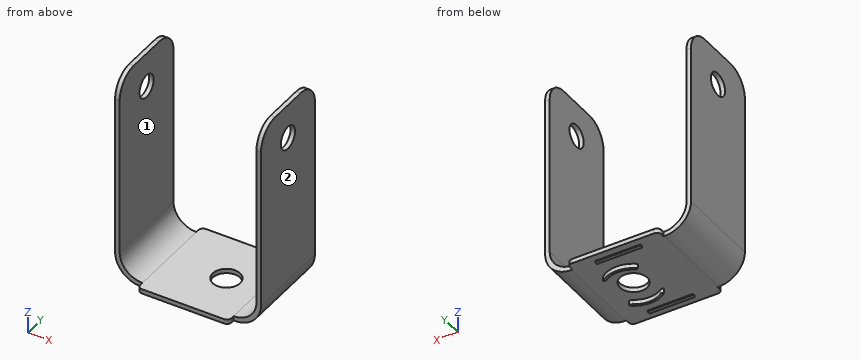
```python
from build123d import *

# Parameters (mm, degrees)
F1_DEPTH  = 38
F3_D      = 12
F5_DEPTH  = 2
F6_R      = 10
F8_DEPTH  = 0.5
F10_DEPTH = 2
F12_D     = 10


with BuildPart() as f1:
    # F0 (on Front) → F1 (new body)
    with BuildSketch(Plane.XZ):
        with BuildLine():
            Line((20, 0), (0, 0))
            Line((0, 0), (-20, 0))
            ThreePointArc((-20, 0), (-27.0710678119, 2.9289321881), (-30, 10))
            Line((-30, 10), (-30, 90))
            Line((-30, 90), (-32, 90))
            Line((-32, 90), (-32, 9.5))
            ThreePointArc((-32, 9.5), (-28.6317279836, 1.3682720164), (-20.5, -2))
            Line((-20.5, -2), (0, -2))
            Line((0, -2), (20.5, -2))
            ThreePointArc((20.5, -2), (28.6317279836, 1.3682720164), (32, 9.5))
            Line((32, 9.5), (32, 90))
            Line((32, 90), (30, 90))
            Line((30, 90), (30, 10))
            ThreePointArc((30, 10), (27.0710678119, 2.9289321881), (20, 0))
        make_face()
    extrude(amount=F1_DEPTH)

    # F3 (through all)
    with Locations(Plane.XY):
        with Locations((5, -19)):
            Hole(F3_D / 2)

    # F4 (on face) → F5 (join)
    with BuildSketch(Plane(origin=(0, 0, -2), x_dir=(1, 0, 0), z_dir=(0, 0, -1))):
        with BuildLine():
            ThreePointArc((-1, 28.2195444573), (5, 30), (11, 28.2195444573))
            ThreePointArc((11, 28.2195444573), (11.8405728739, 27.8759539642), (12.6811457479, 28.2195444573))
            ThreePointArc((12.6811457479, 28.2195444573), (5, 31), (-2.6811457479, 28.2195444573))
            ThreePointArc((-2.6811457479, 28.2195444573), (-1.8405728739, 27.8759539642), (-1, 28.2195444573))
        make_face()
        with BuildLine():
            ThreePointArc((11, 9.7804555427), (5, 8), (-1, 9.7804555427))
            ThreePointArc((-1, 9.7804555427), (-1.8405728739, 10.1240460358), (-2.6811457479, 9.7804555427))
            ThreePointArc((-2.6811457479, 9.7804555427), (5, 7), (12.6811457479, 9.7804555427))
            ThreePointArc((12.6811457479, 9.7804555427), (11.8405728739, 10.1240460358), (11, 9.7804555427))
        make_face()
    extrude(amount=F5_DEPTH)

    # F6
    f6_edges = [f1.edges().sort_by_distance(p)[0] for p in [
        (-31, -38, 90),
        (31, -38, 90),
        (-31, 0, 90),
        (31, 0, 90),
    ]]
    fillet(f6_edges, radius=F6_R)

    # F7 (on face) → F8 (join)
    with BuildSketch(Plane(origin=(0, 0, -2), x_dir=(1, 0, 0), z_dir=(0, 0, -1))):
        Polygon((10, 36.75), (10, 37.5), (10, 38.25), (-10, 38.25), (-10, 36.75), align=None)
        Polygon((10, -0.25), (10, 0.5), (10, 1.25), (-10, 1.25), (-10, -0.25), align=None)
    extrude(amount=F8_DEPTH)

    # F9 (on face) → F10 (join)
    with BuildSketch(Plane.XY):
        with BuildLine():
            Line((-20, 1.5), (-20, 0))
            Line((-20, 0), (20, 0))
            Line((20, 0), (20, 1.5))
            ThreePointArc((20, 1.5), (19.4142135624, 2.9142135624), (18, 3.5))
            Line((18, 3.5), (-18, 3.5))
            ThreePointArc((-18, 3.5), (-19.4142135624, 2.9142135624), (-20, 1.5))
        make_face()
        with BuildLine():
            ThreePointArc((18, -41.5), (19.4142135624, -40.9142135624), (20, -39.5))
            Line((20, -39.5), (20, -38))
            Line((20, -38), (-20, -38))
            Line((-20, -38), (-20, -39.5))
            ThreePointArc((-20, -39.5), (-19.4142135624, -40.9142135624), (-18, -41.5))
            Line((-18, -41.5), (18, -41.5))
        make_face()
    extrude(amount=-F10_DEPTH)

    # F12 (through all)
    with Locations(Plane.YZ.offset(32)):
        with Locations((-19, 75)):
            Hole(F12_D / 2)


solid = f1.part
```
Source: CAD feature listing. Evaluate the final solid. Frame: model axes, mm. Face numbers are marked on the shaded views. A direction names the side the tool comes from. Round coordinates to 2 decimals unless told otherwise and drop trailing zeros. Order: outer loops, then holes, each group sorted by start corner. A loop starts at its lowest first (then second) coordinate and runs counter-clockwise, first axis right, second up. Notation, with made-up numbers: (67.5, -26.5) -> (117.5, -26.5) arc R30 cw to (117.5, 8.5) -> close; hole circle Ø2 at (-18, 85.5). An arc over 180 degrees is marked (long way). One line per item, written item: value. Start each with the question number.
Q1. Section query B-B (z = 57). Return the cut outline in (x, y).
Q2. Section query C-C (x = 5). Return the cut outline in (y, z).
Q3. Section query A-A (y = -19). Return the cut outline in (x, z), plus the area to 3 significant figures.
Q4. Section query D-D (z = 75). Return the cut outline in (x, y).
Q5. Material intervals for probe 1 along X at (y, z) = (-15, 35.5); probe 2 along Z at (x, y) = (-8, -13); probe 3 along X at (y, z) = (-34.5, 1.5), sorted ascending.
Q6. Access query for the marked faces 1 and 2. Directions: +Z, -Z, +X, -X, +Y, -Y. A direction counts if a zero-diameter tool reaches every point of the face in a straight line with its end or side. Return the directions, or none.
Q7. Pin query (flat end, axial travel): pin 1 (4 mm diameter, centred on x = -4, y = -18, fed in from -Z); pin 2 (1.6 mm diameter, centred on y = -38.5, z = -0.5, fed in from -X); pin 3 (12 mm diameter, centred on x = -6.5, y = -14, fed in from +Z); pin 4 (9 mm diameter, centred on y = -19, z = 75, fed in from -X). Return the tip coordinate at first contact, or that it passes through.
Findings below:
1. outline: (-32, -38) -> (-30, -38) -> (-30, 0) -> (-32, 0) -> close; (30, -38) -> (32, -38) -> (32, 0) -> (30, 0) -> close
2. outline: (-41.5, -2) -> (-38.25, -2) -> (-38.25, -2.5) -> (-36.75, -2.5) -> (-36.75, -2) -> (-31, -2) -> (-31, -4) -> (-30, -4) -> (-30, -2) -> (-25, -2) -> (-25, 0) -> (-41.5, 0) -> close; (-13, -2) -> (-8, -2) -> (-8, -4) -> (-7, -4) -> (-7, -2) -> (-1.25, -2) -> (-1.25, -2.5) -> (0.25, -2.5) -> (0.25, -2) -> (3.5, -2) -> (3.5, 0) -> (-13, 0) -> close
3. outline: (-32, 9.5) arc R11.5 ccw to (-20.5, -2) -> (-1, -2) -> (-1, 0) -> (-20, 0) arc R10 cw to (-30, 10) -> (-30, 70) -> (-32, 70) -> close; (-32, 80) -> (-30, 80) -> (-30, 90) -> (-32, 90) -> close; (11, -2) -> (20.5, -2) arc R11.5 ccw to (32, 9.5) -> (32, 70) -> (30, 70) -> (30, 10) arc R10 cw to (20, 0) -> (11, 0) -> close; (30, 80) -> (32, 80) -> (32, 90) -> (30, 90) -> close
3. area: 410 mm²
4. outline: (-32, -38) -> (-30, -38) -> (-30, -24) -> (-32, -24) -> close; (-32, -14) -> (-30, -14) -> (-30, 0) -> (-32, 0) -> close; (30, -38) -> (32, -38) -> (32, -24) -> (30, -24) -> close; (30, -14) -> (32, -14) -> (32, 0) -> (30, 0) -> close
5. probe 1: -32 to -30, 30 to 32
5. probe 2: -2 to 0
5. probe 3: -28.76 to -25.27, 25.27 to 28.76
6. face 1: +Z, +Y, -Y
6. face 2: +Z, -Z, +X, +Y, -Y
7. pin 1: z = -2
7. pin 2: x = -27.16
7. pin 3: z = 0
7. pin 4: through
